Design review of the part shown in the three views and the two pictorial views. Dimensions are in mm from the part's minimum x, y and z. A direction names the side the tool comes from. Give positions to 0.01 mm unless a question says otherwise; leave off trailing zeros. Write each loop counter-clockwise with the first axis right and the second up, starting at its lowest first coordinate (ties: lowest second). Pieces come first, ordered by that corner, then holes.
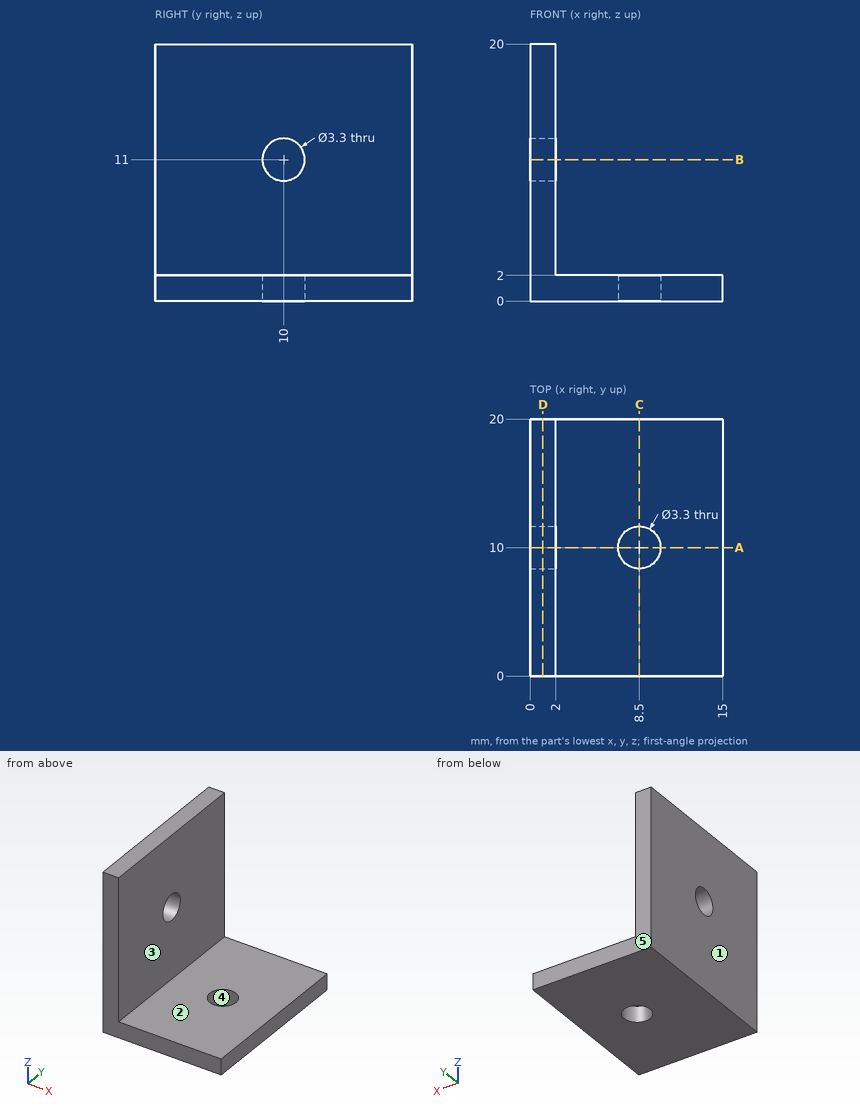
(1) Consider section B-B, the plane z = 11. Give the boundary of the cut face in (x, y).
Resolved:
outline: (0, 0) - (2, 0) - (2, 8.35) - (0, 8.35) - close; (0, 11.65) - (2, 11.65) - (2, 20) - (0, 20) - close
(2) Mouldability with a two-part tool opening along X and no side actions: class the marked faces 3, 4 and 5 as pulls with the +X half, pulls with the -X half, needs draft (parallel to the pull), parting line crosses it, or undercut.
Resolved:
face 3: pulls with the +X half
face 4: undercut
face 5: needs draft
(3) Tool access review of the marked faces 1 and 2: name each direction out of +Z, -Z, +X, -X, +Y, -Y from which nothing blocks a thin tool from reaching the whole face with its end or side.
Resolved:
face 1: +Z, -Z, -X, +Y, -Y
face 2: +Z, +X, +Y, -Y
(4) Consider section A-A, the plane y = 10. Give the boundary of the cut face in (x, z).
Resolved:
outline: (0, 0) - (6.85, 0) - (6.85, 2) - (2, 2) - (2, 9.35) - (0, 9.35) - close; (0, 12.65) - (2, 12.65) - (2, 20) - (0, 20) - close; (10.15, 0) - (15, 0) - (15, 2) - (10.15, 2) - close
(5) Consider section D-D, the plane x = 1. Give the boundary of the cut face in (y, z).
Resolved:
outline: (0, 0) - (20, 0) - (20, 20) - (0, 20) - close; hole circle Ø3.3 at (10, 11)
(6) Consider section C-C, the plane x = 8.5. Give the boundary of the cut face in (y, z), then the cut area to 3 significant figures.
Resolved:
outline: (0, 0) - (8.35, 0) - (8.35, 2) - (0, 2) - close; (11.65, 0) - (20, 0) - (20, 2) - (11.65, 2) - close
area: 33.4 mm2
(7) Clearance check with flat-ended pins moving along their axes: P1, Ø12, axis at y = 13, z = 11, coming from the +X side; P2, Ø5.5, axis at x = 8.5, y = 10, coming from the +Z side. State where each tip first meets the part, or that it passes through.
Resolved:
P1: stops at x = 2
P2: stops at z = 2
(8) To check wall thickness, follow L1, parallel to Y at x = 8.5, z = 1.45; L2, parallel to Z at x = 1.4, y = 10; L3, parallel to Z at x = 7.5, y = 16.5. State the ranges of each line that lie inside material, in increasing order.
Resolved:
L1: y = 0 to 8.35, 11.65 to 20
L2: z = 0 to 9.35, 12.65 to 20
L3: z = 0 to 2
